Here's the drawing with two shaded views (mm, measured from the low corner). I have some questions. Coordinates: 2 decimals unless noted, no trailing zeros. Order: outer loops, then holes, each group sorted by start corner. A loop starts at its lowest first (then second) coordinate and runs counter-clockwise, first axis right, second up. Notation, with made-up numbers: (-21, 5.5) - (-16, 5.5) arc R15 cw to (-16, 11.5) - close; hole circle Ø4 at (14.25, 55). An arc over 180 degrees is marked (long way). One line per item, written item: value. Start each with the question number.
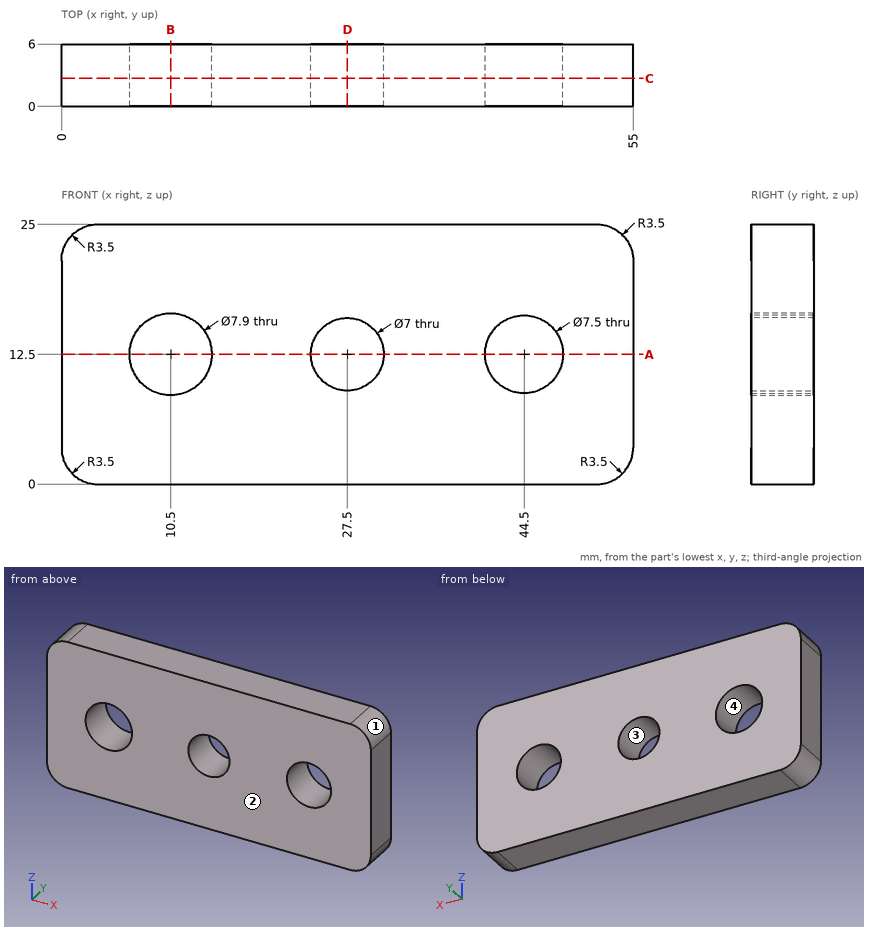
Q1. I'm going to push a flat-ended pin straight in: pin 1 (4.5 mm diameter, centred on x = 44.5, z = 12.5, fed in from +Y). Where does the tip first touch, or does it pass through?
Q2. If I drill on L1, parallel to X at y = 4.1, z = 12.5; L2, parallel to X at y = 1.7, z = 14; L3, parallel to X at y = 4.05, z = 22.5, over which ranges is the centre line in solid material (lowest first)?
Q3. I want a section at D-D on x = 27.5. Please give me the cut outline in (y, z).
Q4. I want a section at C-C on y = 2.7. Please give me the cut outline in (x, z).
Q5. I want a section at B-B on x = 10.5. Please give me the cut outline in (y, z).
Q6. I want a section at A-A on z = 12.5. Please give me the cut outline in (x, y).
Q7. We'd pull the mould along Z, two halves only. Please class the marked faces 1, 2, 3 and 4: +Z half, -Z half, draft (parallel to the pull), parting line (faces both ways), or undercut.
Values follow:
1. pin 1: passes through
2. L1: x = 0 to 6.55, 14.45 to 24, 31 to 40.75, 48.25 to 55
2. L2: x = 0 to 6.85, 14.15 to 24.34, 30.66 to 41.06, 47.94 to 55
2. L3: x = 0.15 to 54.85
3. outline: (0, 0) - (6, 0) - (6, 9) - (0, 9) - close; (0, 16) - (6, 16) - (6, 25) - (0, 25) - close
4. outline: (0, 3.5) arc R3.5 ccw to (3.5, 0) - (51.5, 0) arc R3.5 ccw to (55, 3.5) - (55, 21.5) arc R3.5 ccw to (51.5, 25) - (3.5, 25) arc R3.5 ccw to (0, 21.5) - close; hole circle Ø7.9 at (10.5, 12.5); hole circle Ø7 at (27.5, 12.5); hole circle Ø7.5 at (44.5, 12.5)
5. outline: (0, 0) - (6, 0) - (6, 8.55) - (0, 8.55) - close; (0, 16.45) - (6, 16.45) - (6, 25) - (0, 25) - close
6. outline: (0, 0) - (6.55, 0) - (6.55, 6) - (0, 6) - close; (14.45, 0) - (24, 0) - (24, 6) - (14.45, 6) - close; (31, 0) - (40.75, 0) - (40.75, 6) - (31, 6) - close; (48.25, 0) - (55, 0) - (55, 6) - (48.25, 6) - close
7. face 1: +Z half
7. face 2: draft
7. face 3: undercut
7. face 4: undercut
